Work out the finished part from the listing and answer in its coordinate system (mm). Face numbers are marked on the shaded views. A direction names the side the tool comes from. Give positions to 0.01 mm unless a question says otherwise; leave off trailing zeros. Loops run counter-clockwise (first coordinate to the right, second up) from the corner with the lowest first, then second, coordinate; pieces in that order, holes last. Notation, with made-up numbers: (54, 41) - (60, 41) arc R17 ccw to (60, 45) - close; hole circle Ø1 at (47, -4). An arc over 180 degrees is marked (long way). One line per item, written item: value.
Autodesk Inventor part; units mm, degrees
ref_plane "YZ Plane" through (0, 0, 0) normal (1, 0, 0) x (0, 1, 0)
ref_plane "XZ Plane" through (0, 0, 0) normal (0, 1, 0) x (-1, 0, 0)
ref_plane "XY Plane" through (0, 0, 0) normal (0, 0, 1) x (1, 0, 0)
sketch "スケッチ1" plane through (0, 0, 0) normal (1, 0, 0) x (0, 1, 0)
  circle A0 centre (0, 0) radius 3.5
  dimension "d0" = 7
extrude "押し出し1" add sketch "スケッチ1" along normal blind 3.5
sketch "スケッチ2" plane through (3.5, 0, 0) normal (1, 0, 0) x (0, 0, -1)
  circle A0 centre (0, 0) radius 2.675
  dimension "d3" = 5.35
extrude "押し出し2" cut sketch "スケッチ2" against normal blind 2.1
sketch "スケッチ3" plane through (0, 0, 0) normal (-1, 0, 0) x (0, 0, 1)
  circle A0 centre (0, 0) radius 2.5
  dimension "d6" = 5
extrude "押し出し3" add sketch "スケッチ3" along normal blind 1.3
sketch "スケッチ4" plane through (-1.3, 0, 0) normal (-1, 0, 0) x (0, 0, 1)
  circle A0 centre (0, 0) radius 1.5
  dimension "d9" = 3
extrude "押し出し4" cut sketch "スケッチ4" against normal through all
chamfer "面取り4" distance 1 angle 45 1 edges at (0, -3.5, 0)
chamfer "面取り5" distance 0.5 angle 45 1 edges at (-1.3, 0, -2.5)
properties part number "MagnetMounter"
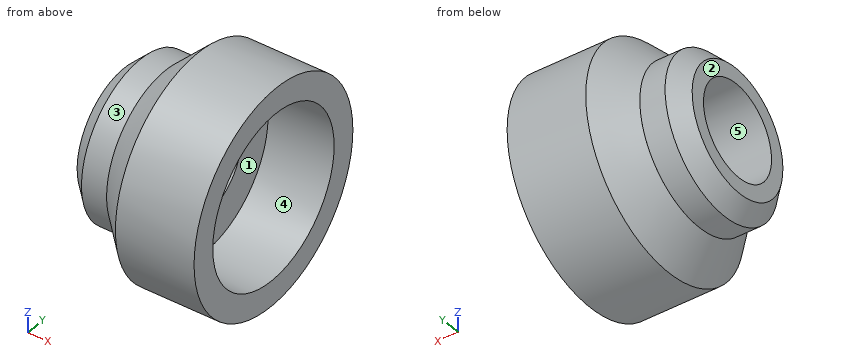
1. Section C-C (x = -0.4) is taken. Write down the section's boundary in (y, z).
Output:
outline: circle Ø5 at (0, 0); hole circle Ø3 at (0, 0)
2. A flat-ended cylindrical pin translates along its axis: pin 1 Ø4 at (y, z) = (1, 2) entering from +X. Find the tip coordinate at first contact, or state that the pin passes through.
Output:
pin 1: stops at x = 3.5
3. Section D-D (x = 2) is taken. Write down the section's boundary in (y, z) (3 decimals).
Output:
outline: circle Ø7 at (0, 0); hole circle Ø5.35 at (0, 0)
4. For the marked faces 4 and 5, determine the directions among +Z, -Z, +X, -X, +Y, -Y from which every point of the face is accessible in a straight line to the end or side of a thin tool.
Output:
face 4: +X
face 5: +X, -X
5. Find the intervals of material crossed by line 1 along Y through (x, z) = (-0.05, 0); line 2 along Y through (x, z) = (0.8, 0); line 3 along Z through (x, y) = (2.4, -0.75), in increasing order.
Output:
line 1: y = -2.5 to -1.5, 1.5 to 2.5
line 2: y = -3.3 to -1.5, 1.5 to 3.3
line 3: z = -3.42 to -2.57, 2.57 to 3.42
6. The mould has two halves that part along Z. Classify the marked faces 1, 2 and 3: released by +Z, released by -Z, zero draft, split by the parting line, or undercut.
Output:
face 1: undercut
face 2: zero draft
face 3: split by the parting line
